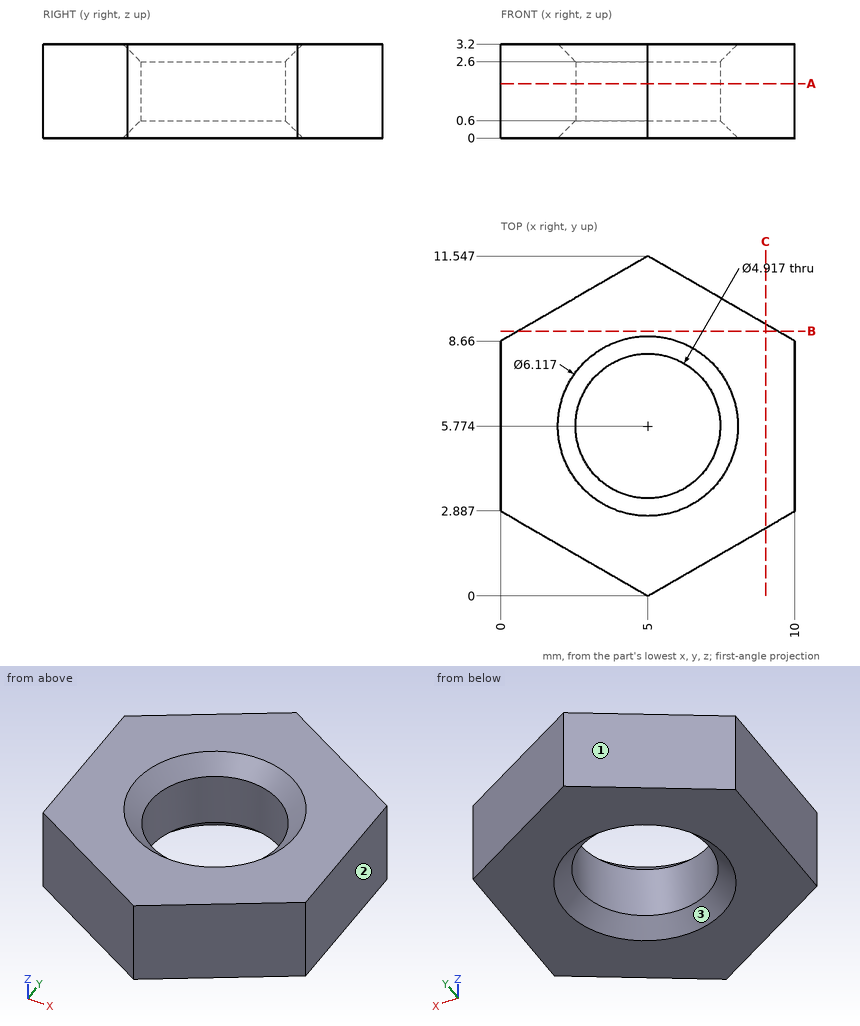
Can you work these out from the drawing? Everything is in mm from the part's minimum corner. Coordinates: 2 decimals unless noted, no trailing zeros. Loops run counter-clockwise (first coordinate to the right, second up) from the corner with the lowest first, then second, coordinate; pieces in that order, holes last. Notation, with made-up numbers: (-20, 34) - (19, 34) arc R20 cw to (19, 50) - close; hole circle Ø10 at (62.5, 6.5). An arc over 180 degrees is marked (long way). Use a Markdown table: item, result.
Item 1: If I drill on probe 1 along X at (y, z) = (4.25, 2.2); probe 2 along X at (y, z) = (5.75, 2.4); probe 3 along X at (y, z) = (2, 0.75) (1 decimal), over which ranges is the centre line in solid material (lowest first)? Write a range as from..to.
Numbers:
| item | result |
|---|---|
| probe 1 | x = 0..3.07, 6.93..10 |
| probe 2 | x = 0..2.54, 7.46..10 |
| probe 3 | x = 1.5..8.5 |
Item 2: We'd pull the mould along Y, two halves only. Please class the marked faces 1, 2 and 3: released by +Y, released by -Y, zero draft, split by the parting line, or undercut.
Numbers:
| item | result |
|---|---|
| face 1 | released by +Y |
| face 2 | zero draft |
| face 3 | undercut |
Item 3: I want a section at B-B on y = 9. Please give me the cut outline in (x, z).
Numbers:
| item | result |
|---|---|
| outline | (0.59, 0) - (9.41, 0) - (9.41, 3.2) - (0.59, 3.2) - close |
Item 4: Will this pin go through, and if not, where does the flat tip stop? pin 1 (1 mm diameter, centred on x = 7.5, z = 2, fed in from -Y) (1 decimal).
Numbers:
| item | result |
|---|---|
| pin 1 | stops at y = 1.2 |
Item 5: I want a section at C-C on x = 9. Please give me the cut outline in (y, z).
Numbers:
| item | result |
|---|---|
| outline | (2.31, 0) - (9.24, 0) - (9.24, 3.2) - (2.31, 3.2) - close |
Item 6: I want a section at A-A on z = 1.85. Please give me the cut outline in (x, y) (1 decimal).
Numbers:
| item | result |
|---|---|
| outline | (0, 2.9) - (5, 0) - (10, 2.9) - (10, 8.7) - (5, 11.5) - (0, 8.7) - close; hole circle Ø4.9 at (5, 5.8) |
